Geometry check sheet. Reference: drawing and pictorial views, mm from the part's lowest x, y, z. Coordinates: 2 decimals unless noted, no trailing zeros. Loops run counter-clockwise (first coordinate to the right, second up) from the corner with the lowest first, then second, coordinate; pieces in that order, holes last. Notation, with made-up numbers: M -27,-25.5 L 6,-25.5 A22 cw 6,-12.5 Z; hole C 50,-18.5 d5. An arc over 180 degrees is marked long. Write item = value, one per line. Start each with the question number.
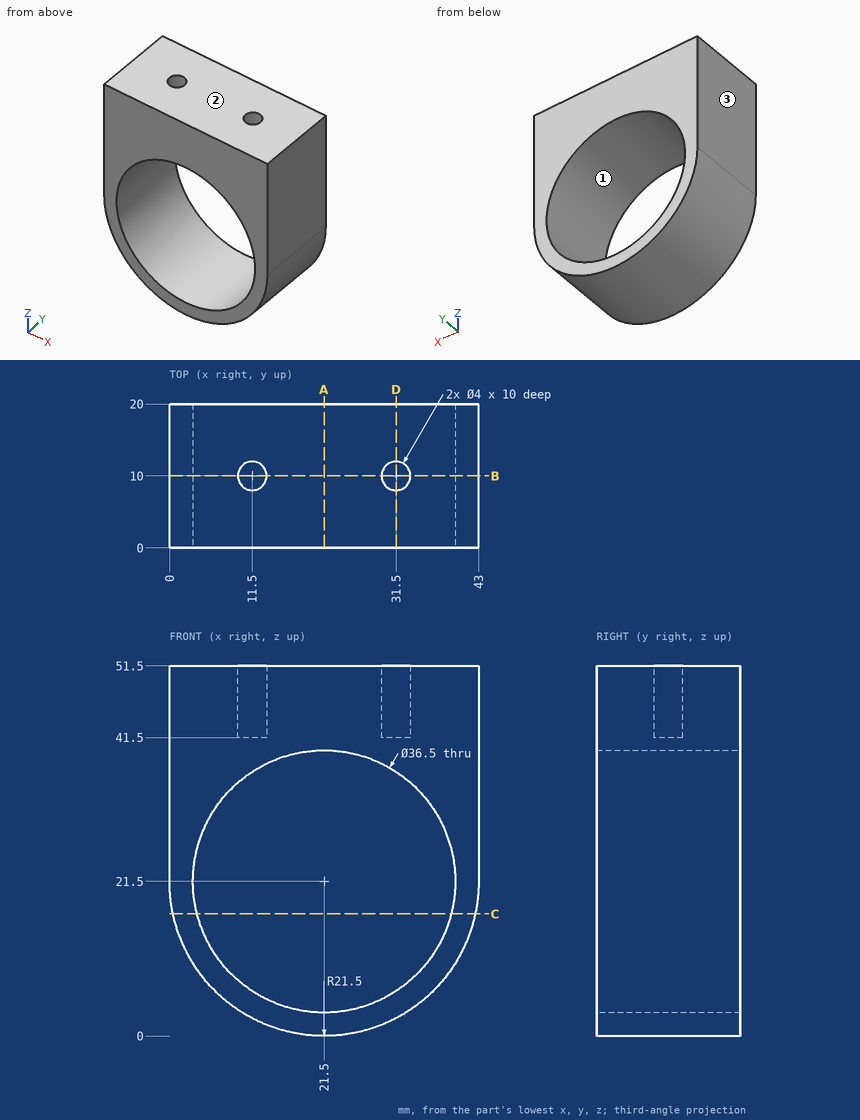
Q1. Scan lines: L1, parallel to Y at x = 31.5, z = 46.5; L2, parallel to Z at x = 27.5, y = 3.75; L3, parallel to Z at x = 12, y = 7.25. Record each from-to range of solid material in increasing order. Write a range as [from, to].
Q2. Sectioned sample at D-D on x = 31.5. Record the cut outline in (y, z).
Q3. Gauge pin test, flat ends, axial feed: pin 1 (4 mm diameter, centred on x = 8.5, y = 13.5, fed in from -Z); pin 2 (5 mm diameter, centred on x = 11.5, y = 10, fed in from -Z); pin 3 (1.5 mm diameter, centred on x = 24.5, y = 17.5, fed in from -Z). Record the tip position at first contact, or that the pin passes through.
Q4. Sectioned sample at B-B on y = 10. Record the cut outline in (x, z), plus the area to 3 significant figures.
Q5. Sectioned sample at C-C on z = 17. Record the cut outline in (x, y), plus the area to 3 significant figures.
Q6. Sectioned sample at A-A on x = 21.5. Record the cut outline in (y, z).
Q7. Mould release check, pull along Z, two halves, no side actions. Record for the marked faces 1, 2 and 3: +Z half, -Z half, draft (parallel to the pull), parting line (faces both ways), or undercut.
Solutions:
q1.L1 = [0, 8], [12, 20]
q1.L2 = [0.85, 4.26], [38.74, 51.5]
q1.L3 = [2.21, 5.92], [37.08, 51.5]
q2.outline = M 0,2.47 L 20,2.47 L 20,6.23 L 0,6.23 Z; M 0,36.77 L 20,36.77 L 20,51.5 L 12,51.5 L 12,41.5 L 8,41.5 L 8,51.5 L 0,51.5 Z
q3.pin_1 = 3.03
q3.pin_2 = 1.35
q3.pin_3 = 0.12
q4.outline = M 0,21.5 A21.5 ccw 43,21.5 L 43,51.5 L 33.5,51.5 L 33.5,41.5 L 29.5,41.5 L 29.5,51.5 L 13.5,51.5 L 13.5,41.5 L 9.5,41.5 L 9.5,51.5 L 0,51.5 Z; hole C 21.5,21.5 d36.5
q4.area = 890 mm²
q5.outline = M 0.48,0 L 3.81,0 L 3.81,20 L 0.48,20 Z; M 39.19,0 L 42.52,0 L 42.52,20 L 39.19,20 Z
q5.area = 133 mm²
q6.outline = M 0,0 L 20,0 L 20,3.25 L 0,3.25 Z; M 0,39.75 L 20,39.75 L 20,51.5 L 0,51.5 Z
q7.face_1 = undercut
q7.face_2 = +Z half
q7.face_3 = draft
